Verification items for the finished model (mm, model axes). Face numbers are marked on the shaded views. A direction names the side the tool comes from. Round coordinates to 2 decimals unless told otherwise and drop trailing zeros. Order: outer loops, then holes, each group sorted by start corner. A loop starts at its lowest first (then second) coordinate and runs counter-clockwise, first axis right, second up. Notation, with made-up numbers: (11.25, -10) -> (24.25, -10) arc R21 ccw to (24.25, 26) -> close; hole circle Ø8 at (-24.75, 13). An arc over 180 degrees is marked (long way). Return JSON: item names as keys, results as strings. Group by question number.
Item 1: Access from +Z, -Z, +X, -X, +Y, -Y to the whole of each face (thin tool, end or side, straight path). Record for the marked faces 1 and 2.
Item 2: Sectioned sample at B-B on x = 0. Record the cut outline in (y, z), plus the area to 3 significant figures.
Item 3: Sectioned sample at A-A on z = 2.75. Record the cut outline in (x, y).
Item 4: Scan lines: probe 1 along X at (y, z) = (12.5, 3.7); probe 2 along X at (y, z) = (20.5, 0.35); probe 3 along Y at (x, z) = (43, 2.2). Record each from-to range of solid material in increasing order. Write a range as from..to.
Item 5: Sectioned sample at D-D on y = -17. Record the cut outline in (x, z), plus the area to 3 significant figures.
Item 6: Sectioned sample at C-C on y = -30. Record the cut outline in (x, z), plus the area to 3 significant figures.
Item 7: Depth check by flat-ended pin: pin 1 Ø5.5 at (x, y) = (26.06, 20.38) entering from -Z; pin 2 Ø8 at (x, y) = (-35, 21) entering from +Z. Enter the tip coordinate at first touch or a pass-through.
```python
from build123d import *

# Parameters (mm, degrees)
F0_W     = 106.79
F0_H     = 70.9
F0_R     = 2.05
F1_DEPTH = 2
F0_W_2   = 116.79
F0_H_2   = 80.9
F2_DEPTH = 4


with BuildPart() as f1:
    # F0 (on Top) → F1 (new body)
    with BuildSketch(Plane.XY):
        with Locations((-10.0916011143, -8.5682209864)):
            Rectangle(F0_W, F0_H)
        with Locations((-47.0616011143, -37.5182209864)):
            Circle(F0_R, mode=Mode.SUBTRACT)
        with Locations((26.2383988857, -37.5182209864)):
            Circle(F0_R, mode=Mode.SUBTRACT)
        with Locations((-47.2416011143, 20.3817790136)):
            Circle(F0_R, mode=Mode.SUBTRACT)
        with BuildLine():
            Line((23.3033988857, -22.5132511556), (-43.4866011143, -22.5132511556))
            ThreePointArc((-43.4866011143, -22.5132511556), (-58.4866011143, -7.5132511556), (-43.4866011143, 7.4867488444))
            Line((-43.4866011143, 7.4867488444), (23.3033988857, 7.4867488444))
            ThreePointArc((23.3033988857, 7.4867488444), (38.3033988857, -7.5132511556), (23.3033988857, -22.5132511556))
        make_face(mode=Mode.SUBTRACT)
        with Locations((26.0583988857, 20.3817790136)):
            Circle(F0_R, mode=Mode.SUBTRACT)
    extrude(amount=F1_DEPTH)

    # F0 (on Top) → F2 (join)
    with BuildSketch(Plane.XY):
        with Locations((-10.0916011143, -8.5682209864)):
            Rectangle(F0_W_2, F0_H_2)
        with Locations((-10.0916011143, -8.5682209864)):
            Rectangle(F0_W, F0_H, mode=Mode.SUBTRACT)
    extrude(amount=F2_DEPTH)


solid = f1.part
```
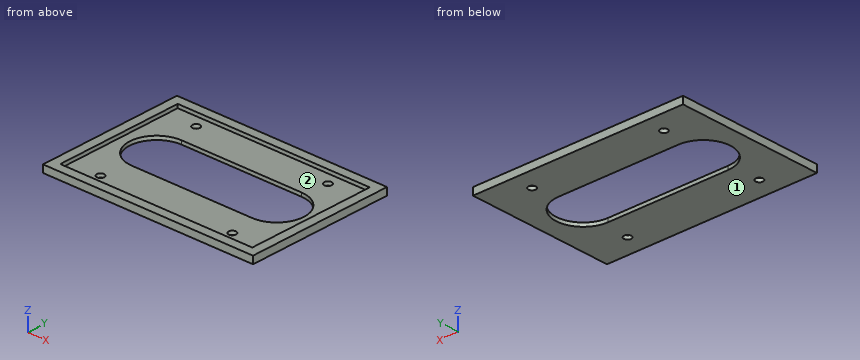
Recorded:
{
 "1": {"face 1": "-Z, +X, -X, +Y, -Y", "face 2": "+Z"},
 "2": {"outline": "(-49.02, 0) -> (-22.51, 0) -> (-22.51, 2) -> (-44.02, 2) -> (-44.02, 4) -> (-49.02, 4) -> close; (7.49, 0) -> (31.88, 0) -> (31.88, 4) -> (26.88, 4) -> (26.88, 2) -> (7.49, 2) -> close", "area": "122 mm²"},
 "3": {"outline": "(-68.49, -49.02) -> (48.3, -49.02) -> (48.3, 31.88) -> (-68.49, 31.88) -> close; hole (-63.49, -44.02) -> (43.3, -44.02) -> (43.3, 26.88) -> (-63.49, 26.88) -> close"},
 "4": {"probe 1": "-68.49..-63.49, 43.3..48.3", "probe 2": "-68.49..-49.29, -45.2..24.01, 28.1..48.3", "probe 3": "-49.02..-44.02, 26.88..31.88"},
 "5": {"outline": "(-68.49, 0) -> (-55.11, 0) -> (-55.11, 2) -> (-63.49, 2) -> (-63.49, 4) -> (-68.49, 4) -> close; (34.92, 0) -> (48.3, 0) -> (48.3, 4) -> (43.3, 4) -> (43.3, 2) -> (34.92, 2) -> close", "area": "73.5 mm²"},
 "6": {"outline": "(-68.49, 0) -> (48.3, 0) -> (48.3, 4) -> (43.3, 4) -> (43.3, 2) -> (-63.49, 2) -> (-63.49, 4) -> (-68.49, 4) -> close", "area": "254 mm²"},
 "7": {"pin 1": "z = 0", "pin 2": "z = 2"}
}
